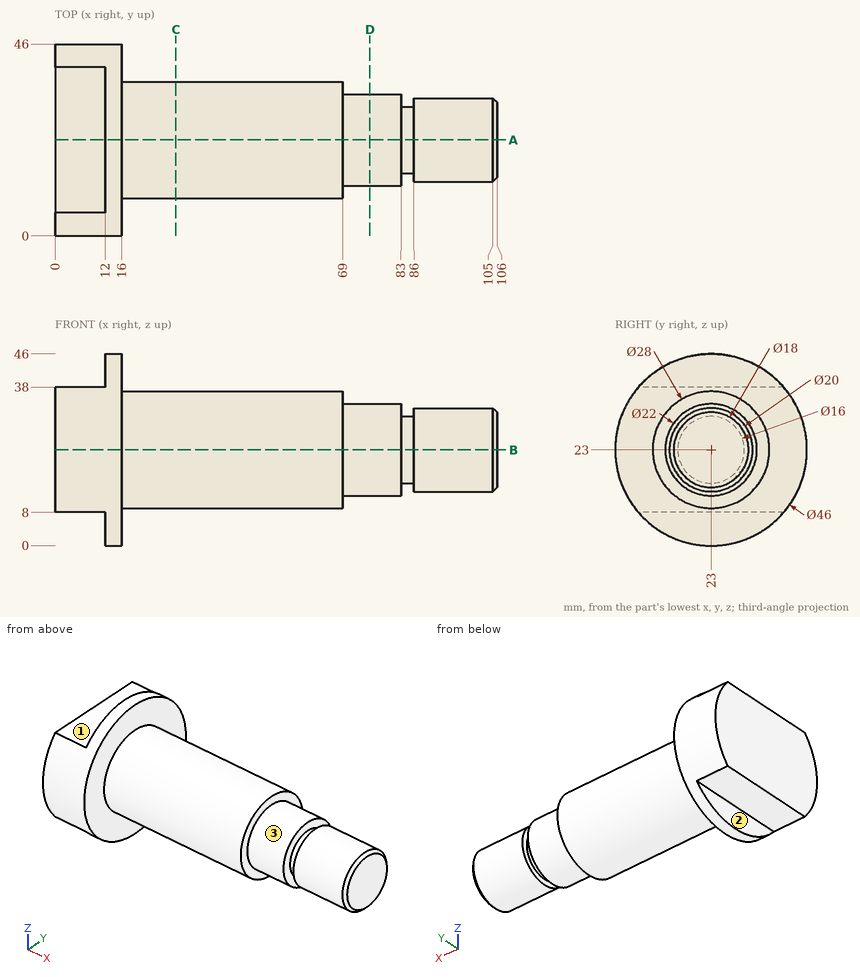
Can you work these out from the drawing? Everything is in mm from the part's minimum corner. A direction names the side the tool comes from. Give positions to 0.01 mm unless a question says otherwise; leave off trailing zeros. Loops run counter-clockwise (first coordinate to the right, second up) from the corner with the lowest first, then second, coordinate; pieces in that order, holes last. Notation, with made-up numbers: (9, 42.25) - (15, 42.25) arc R24 cw to (15, 71.25) - close; hole circle Ø9 at (70, 36.25). An arc over 180 degrees is marked (long way). Use one line per item in the form item = value.
1. I need wall thicknesses on probe 1 along X at (y, z) = (26, 3); probe 2 along X at (y, z) = (13, 9.5); probe 3 along Y at (x, z) = (98, 23.5). Which ranges of each line are inside material? Lowest first, please.
Response values:
probe_1 = 12 to 16
probe_2 = 0 to 16
probe_3 = 13.01 to 32.99
2. I'm going to push flat-ended pins straight in: pin 1 Ø3.5 at (x, y) = (6.5, 21.5) entering from -Z; pin 2 Ø10 at (x, y) = (20.5, 17) entering from -Z; pin 3 Ø9.5 at (x, y) = (6.5, 23.5) entering from +Z. Where does each tip first touch, or does it pass through?
Response values:
pin_1 = 8
pin_2 = 0.32
pin_3 = 38
3. I want a section at A-A (y = 23). Please give me the cut outline in (x, z).
Response values:
outline = (0, 8) - (12, 8) - (12, 0) - (16, 0) - (16, 9) - (69, 9) - (69, 12) - (83, 12) - (83, 15) - (86, 15) - (86, 13) - (105, 13) - (106, 14) - (106, 32) - (105, 33) - (86, 33) - (86, 31) - (83, 31) - (83, 34) - (69, 34) - (69, 37) - (16, 37) - (16, 46) - (12, 46) - (12, 38) - (0, 38) - close
4. On a 3-axis mill with a long thin cutter (end or side, diameter ignored), from which of +Z, -Z, +X, -X, +Y, -Y can I reach the whole of each face in a straight line? I mean the marked faces 1, 2 and 3. Say none if no direction works.
Response values:
face_1 = +Z, -X, +Y, -Y
face_2 = -Z, -X, +Y, -Y
face_3 = +X
5. I want a section at D-D (x = 75.5). Please give me the cut outline in (y, z).
Response values:
outline = circle Ø22 at (23, 23)
6. I want a section at C-C (x = 29). Please give me the cut outline in (y, z).
Response values:
outline = circle Ø28 at (23, 23)
7. I want a section at B-B (z = 23). Please give me the cut outline in (x, y).
Response values:
outline = (0, 0) - (16, 0) - (16, 9) - (69, 9) - (69, 12) - (83, 12) - (83, 15) - (86, 15) - (86, 13) - (105, 13) - (106, 14) - (106, 32) - (105, 33) - (86, 33) - (86, 31) - (83, 31) - (83, 34) - (69, 34) - (69, 37) - (16, 37) - (16, 46) - (0, 46) - close
